Autodesk Inventor part; units mm, degrees
ref_plane "YZ Plane" through (0, 0, 0) normal (1, 0, 0) x (0, 1, 0)
ref_plane "XZ Plane" through (0, 0, 0) normal (0, 1, 0) x (-1, 0, 0)
ref_plane "XY Plane" through (0, 0, 0) normal (0, 0, 1) x (1, 0, 0)
sketch "Sketch1" plane through (0, 0, 0) normal (0, 0, 1) x (1, 0, 0)
  line L0 (10, 0) -> (35, 0)
  line L1 (35, 0) -> (35, -10)
  line L2 (35, -10) -> (25, -10)
  line L3 (25, -10) -> (25, -30)
  line L4 (25, -30) -> (10, -30)
  line L5 (10, -30) -> (10, 0)
  line L6 (0, 0) -> (0, -47.182838) construction
  dimension "d0" = 10
  dimension "d1" = 20
  dimension "d2" = 35
  dimension "d3" = 10
  dimension "d4" = 10
  dimension "d5" = 0
sketch "Sketch1 outline for Revolution1" plane through (0, 0, 0) normal (0, 0, 1) x (1, 0, 0)
  line L0 (10, 0) -> (10, -30)
  line L1 (35, 0) -> (10, 0)
  line L2 (35, -10) -> (35, 0)
  line L3 (25, -10) -> (35, -10)
  line L4 (25, -30) -> (25, -10)
  line L5 (10, -30) -> (25, -30)
revolve "Revolution1" add sketch "Sketch1 outline for Revolution1" angle 360 about axis through (0, 0, 0) along (0, -1, 0)
sketch "Sketch2" plane through (0, 0, 0) normal (0, 1, 0) x (-1, 0, 0)
  circle A0 centre (0, 0) radius 35
  arc A1 (11.18034, -10) -> (11.18034, 10) centre (0, 0) ccw
  line L0 (11.18034, 10) -> (29.349814, 19.067995)
  circle A2 centre (0, 0) radius 35
  line L1 (11.18034, -10) -> (27.938175, -21.082182)
  arc A3 (27.977577, -21.108239) -> (29.6661, 19.225846) centre (0, 0.265385) ccw
  circle A4 centre (0, 0) radius 10
  dimension "d7" = 30
  dimension "d8" = 60
sketch "Sketch2 outline for Extrusion1" plane through (0, 0, 0) normal (0, 1, 0) x (-1, 0, 0)
  arc A0 (11.18034, 10) -> (11.18034, -10) centre (0, 0) cw
  line L0 (29.349814, 19.067995) -> (11.18034, 10)
  arc A1 (27.938175, -21.082182) -> (29.349814, 19.067995) centre (0, 0) ccw
  line L1 (11.18034, -10) -> (27.938175, -21.082182)
extrude "Extrusion1" add sketch "Sketch2 outline for Extrusion1" along normal blind 5
sketch "Sketch3" plane through (0, 0, 0) normal (0, 1, 0) x (-1, 0, 0)
  circle A0 centre (-30, 0) radius 2.5
  point P0 (0, 0)
  dimension "d11" = 5
  dimension "d12" = 30
sketch "Sketch3 outline for Extrusion2" plane through (0, 0, 0) normal (0, 1, 0) x (-1, 0, 0)
  circle A0 centre (-30, 0) radius 2.5
extrude "Extrusion2" cut sketch "Sketch3 outline for Extrusion2" against normal blind 10
pattern_circular "Circular Pattern1" count 3 over 360 about axis through (0, -15, 0) along (0, -1, 0) of "Extrusion1"
pattern_circular "Circular Pattern2" count 3 over 360 about axis through (0, -15, 0) along (0, -1, 0) of "Extrusion2"
properties part number "P01_Marcos_Uriel_Martinez_Ortiz2" material "Steel ASTM A36"
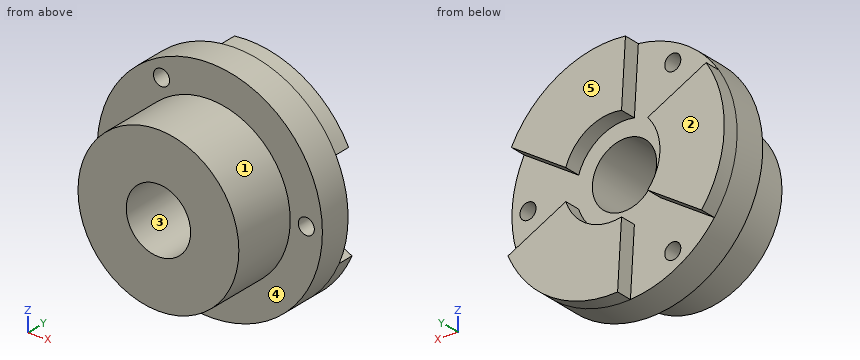
Part model, mm, in its own coordinate system. Face numbers are marked on the shaded views. A direction names the side the tool comes from. Round coordinates to 2 decimals unless told otherwise and drop trailing zeros. Write each loop counter-clockwise with the first axis right and the second up, starting at its lowest first coordinate (ties: lowest second). Pieces come first, ordered by that corner, then holes. Notation, with made-up numbers: (-6.75, -16) - (46.25, -16) arc R29 cw to (46.25, 4) - close; hole circle Ø4 at (-12, 18). An arc over 180 degrees is marked (long way). Use CSV: the item, a comma, the result in double quotes.
Item 1: Tool access for the marked faces 4 and 5: list every direction of +Z, -Z, +X, -X, +Y, -Y with a clear straight run to the whole face (end or side of a thin tool).
Results list:
face 4,"-Y"
face 5,"+Z, -Z, +X, -X, +Y"
Item 2: Wall check: L1, parallel to Z at x = 0, y = -9.25; L2, parallel to Z at x = 0, y = -15.5; L3, parallel to Y at x = -24.5, z = 17.5. Give the ranges that are in metal, low to high.
Results list:
L1,"z = -35 to -10, 10 to 35"
L2,"z = -25 to -10, 10 to 25"
L3,"y = -10 to 0"
Item 3: Slice it at A-A, the plane z = 0. Write the cut outline in (x, y), then the cut area to 3 significant figures.
Results list:
outline,"(-35, -10) - (-25, -10) - (-25, -30) - (-10, -30) - (-10, 0) - (-15, 0) - (-15, 5) - (-35, 5) - close; (10, -30) - (25, -30) - (25, -10) - (27.5, -10) - (27.5, 0) - (10, 0) - close; (32.5, -10) - (35, -10) - (35, 0) - (32.5, 0) - close"
area,"1,150 mm²"
Item 4: Slice it at C-C, the plane z = -27. Write the cut outline in (x, y).
Results list:
outline,"(-22.27, -10) - (-17.28, -10) - (-17.28, 0) - (-22.27, 0) - close; (-12.72, -10) - (22.27, -10) - (22.27, 5) - (-2.32, 5) - (-2.32, 0) - (-12.72, 0) - close"
Item 5: Slice it at B-B, the plane x = 0. Write the cut outline in (y, z), then the cut area to 3 significant figures.
Results list:
outline,"(-30, -25) - (-10, -25) - (-10, -35) - (5, -35) - (5, -15) - (0, -15) - (0, -10) - (-30, -10) - close; (-30, 10) - (0, 10) - (0, 15) - (5, 15) - (5, 35) - (-10, 35) - (-10, 25) - (-30, 25) - close"
area,"1,300 mm²"
Item 6: Flat gauge pins, fed straight in: P1, Ø4, axis at x = -10, y = -15, coming from the -Z side; P2, Ø6.5, axis at x = 30, z = 0, coming from the -Y side; P3, Ø5, axis at x = 1, y = -24.5, coming from the +Z side; P4, Ø4, axis at x = -15, z = -25.98, coming from the -Y side. Where does each tip first touch, or does it go through?
Results list:
P1,"stops at z = -23.69"
P2,"stops at y = -10"
P3,"stops at z = 25"
P4,"passes through"
Item 7: Slice it at D-D, the plane y = -18. Write the cut outline in (x, z), then the cut area to 3 significant figures.
Results list:
outline,"circle Ø50 at (0, 0); hole circle Ø20 at (0, 0)"
area,"1,650 mm²"
Item 8: Pull direction Z, two halves, no side cores. Call the marked faces 1, 2 and 3: pulls with the +Z half, pulls with the -Z half, needs draft (parallel to the pull), parting line crosses it, or undercut.
Results list:
face 1,"parting line crosses it"
face 2,"needs draft"
face 3,"undercut"
